Autodesk Inventor part; units mm, degrees
ref_plane "YZ Plane" through (0, 0, 0) normal (1, 0, 0) x (0, 1, 0)
ref_plane "XZ Plane" through (0, 0, 0) normal (0, 1, 0) x (-1, 0, 0)
ref_plane "XY Plane" through (0, 0, 0) normal (0, 0, 1) x (1, 0, 0)
sketch "Sketch1" plane through (0, 0, 0) normal (0, 0, 1) x (1, 0, 0)
  circle A0 centre (0, 0) radius 16
  dimension "d0" = 32
extrude "Extrusion1" add sketch "Sketch1" against normal blind 10
sketch "Sketch2" plane through (0, 0, -10) normal (0, 0, -1) x (-1, 0, 0)
  line L0 (0, 7) -> (-14.3875, 7)
  circle A0 centre (0, 0) radius 16
  line L1 (0, 7) -> (14.3875, 7)
  arc A1 (-14.3875, 7) -> (14.3875, 7) centre (0, 0) ccw
  dimension "d3" = 7
extrude "Extrusion2" add sketch "Sketch2" along normal blind 33 contours L1 A0 L0 picked at (0.14, -8.2559)
sketch "Sketch3" plane through (0, 0, -43) normal (0, 0, -1) x (-1, 0, 0)
  circle A0 centre (0, 0) radius 16
  dimension "d6" = 32
extrude "Extrusion3" add sketch "Sketch3" along normal blind 10
sketch "Sketch4" plane through (0, 0, -53) normal (0, 0, -1) x (-1, 0, 0)
  circle A0 centre (0, 0) radius 16
  dimension "d9" = 32
extrude "Extrusion4" add sketch "Sketch4" along normal blind 6 draft -45
sketch "Sketch5" plane through (0, 0, -59) normal (0, 0, -1) x (-1, 0, 0)
  circle A0 centre (0, 0) radius 16
  dimension "d12" = 32
extrude "Extrusion5" add sketch "Sketch5" along normal blind 5
sketch "Sketch6" plane through (0, 0, -64) normal (0, 0, -1) x (-1, 0, 0)
  circle A0 centre (0, 0) radius 10
  dimension "d15" = 20
extrude "Extrusion6" add sketch "Sketch6" along normal blind 10
sketch "Sketch7" plane through (0, 0, 0) normal (0, 0, 1) x (1, 0, 0)
  circle A0 centre (0, 0) radius 16
  dimension "d18" = 32
extrude "Extrusion7" add sketch "Sketch7" along normal blind 11 draft -45
sketch "Sketch8" plane through (0, 0, 11) normal (0, 0, 1) x (1, 0, 0)
  circle A0 centre (0, 0) radius 16
  dimension "d21" = 32
extrude "Extrusion8" add sketch "Sketch8" along normal blind 5
sketch "Sketch9" plane through (0, 0, 16) normal (0, 0, 1) x (1, 0, 0)
  circle A0 centre (0, 0) radius 5
  dimension "d24" = 10
extrude "Extrusion9" add sketch "Sketch9" along normal blind 10
sketch "Sketch10" plane through (-14.3875, 7, -10) normal (0, 1, 0) x (1, 0, 0)
  line L0 (0, 0) -> (0, 33)
  line L1 (28.775, 0) -> (28.775, 33)
  circle A0 centre (14.3875, 16.5) radius 2
  point P0 (14.3875, -10)
  dimension "d27" = 4
hole "Hole1" at (0, 7, -26.5) direction (0, -1, 0) diameter 3.242 end through all
properties part number "MMAE 232 Assignment 1_Part 2 - Dylan Tamras"
CAD build for the part. Positions are in the model's coordinates, mm. A direction names the side the tool comes from. Give positions to 0.01 mm unless a question says otherwise; leave off trailing zeros. Order: outer loops, then holes, each group sorted by start corner. A loop starts at its lowest first (then second) coordinate and runs counter-clockwise, first axis right, second up. Notation, with made-up numbers: (-8, 58.25) -> (36, 58.25) arc R33 ccw to (36, 89.25) -> close; hole circle Ø6 at (80, -5.5). An arc over 180 degrees is marked (long way). Return JSON: item names as keys, results as strings.
Q1. Flat gauge pins, fed straight in: pin 1 (3 mm diameter, centred on y = -4.5, z = -52, fed in from +X); pin 2 (6 mm diameter, centred on y = -7, z = -25, fed in from -X); pin 3 (4 mm diameter, centred on y = -2.5, z = -30.5, fed in from -X). Where does each tip first touch, or does it go through?
Working result:
{"pin 1": "x = 15.72", "pin 2": "x = -15.49", "pin 3": "x = -15.99"}
Q2. Saw through at B-B (y = 0). Write the cut outline in (x, z).
Working result:
{"outline": "(-16, -64) -> (-10, -64) -> (-10, -74) -> (10, -74) -> (10, -64) -> (16, -64) -> (16, -59) -> (10, -59) -> (16, -53) -> (16, 0) -> (5, 11) -> (16, 11) -> (16, 16) -> (5, 16) -> (5, 26) -> (-5, 26) -> (-5, 16) -> (-16, 16) -> (-16, 11) -> (-5, 11) -> (-16, 0) -> (-16, -53) -> (-10, -59) -> (-16, -59) -> close; hole circle Ø3.24 at (0, -26.5)"}
Q3. Drill centre lines: line 1 (Z direction, x = 0, y = -3.25); line 2 (X direction, y = -0.5, z = -26.5); line 3 (Z direction, x = -4.5, y = 12). Where is each one in solid material? Low to high.
Working result:
{"line 1": "-74 to -28.12, -24.88 to 26", "line 2": "-15.99 to -1.62, 1.62 to 15.99", "line 3": "-64 to -59, -56.18 to -43, -10 to 3.18, 11 to 16"}
Q4. Saw through at C-C (z = -26.5). Write the cut outline in (x, y).
Working result:
{"outline": "(-14.39, 7) arc R16 ccw to (-1.62, -15.92) -> (-1.62, 7) -> close; (1.62, -15.92) arc R16 ccw to (14.39, 7) -> (1.62, 7) -> close"}
Q5. Saw through at D-D (z = -51). Write the cut outline in (x, y), then the cut area to 3 significant figures.
Working result:
{"outline": "circle Ø32 at (0, 0)", "area": "804 mm²"}
Q6. Mould opens along Z. For faces 6 (the face through (-1.08, 4.88, 20.93)), 7 (the face through (0.2, -10.4, -64)), 8 (the face through (-4.788, 9.205, -58.625)) say: pulls with the +Z half, pulls with the -Z half, needs draft (parallel to the pull), parting line crosses it, or undercut.
Working result:
{"face 6": "needs draft", "face 7": "pulls with the -Z half", "face 8": "undercut"}
Q7. Which spindle directions (+Z, -Z, +X, -X, +Y, -Y) get a long thin tool onto all of the face, cutting with end or side? Do faces 1 (the face through (-4, 4, 16)), 2 (the face through (3, 7, -26)), 3 (the face through (0, 0, 26)), 4 (the face through (2.17, 9.76, -68.93)), 5 (the face through (0.2, -10.4, -59)). Say none if no direction does.
Working result:
{"face 1": "+Z", "face 2": "+X, -X, +Y", "face 3": "+Z, +X, -X, +Y, -Y", "face 4": "-Z", "face 5": "none"}
